Geometry check sheet. Reference: drawing and pictorial views, mm from the part's lowest x, y, z. A direction names the side the tool comes from. Round coordinates to 2 decimals unless told otherwise and drop trailing zeros. Write each loop counter-clockwise with the first axis right and the second up, starting at its lowest first coordinate (ties: lowest second). Pieces come first, ordered by that corner, then holes.
Item 1: Release check for a two-part mould opening along X. For the marked faces 1, 2 and 3 record: pulls with the +X half, pulls with the -X half, needs draft (parallel to the pull), parting line crosses it, or undercut.
Item 2: Section check D-D, the plane z = 16.75. Record the cut outline in (x, y).
Item 3: Section check A-A, the plane z = 9.75. State how many separate pieces and enclosed holes the cut face has, plus the area to 3 significant figures.
Item 4: Section check C-C, the plane x = 16. Record the cut outline in (y, z), plus the area to 3 significant figures.
Item 5: Depth check by flat-ended pin: pin 1 (1.5 mm diameter, centred on x = 11.5, y = 1, fed in from +Z); pin 2 (5.5 mm diameter, centred on x = 9.75, z = 9.75, fed in from -Y); pin 3 (4 mm diameter, centred on x = 2.75, z = 9.75, fed in from -Y). Enter the tip coordinate at first touch or a pass-through.
Item 6: Material ranges on line 1 along Z through (x, y) = (9.75, 4.2); line 2 along Z through (x, y) = (9.75, 3.85); line 3 along Y through (x, z) = (9.5, 12), recorded low to high.
Item 7: Set-up check for the marked faces 4 and 5: record each of +Z, -Z, +X, -X, +Y, -Y from which the full face is reachable in a straight line by a thin tool's end or side.
Item 8: Section check B-B, the plane x = 9. Record the cut outline in (y, z), plus the area to 3 significant figures.
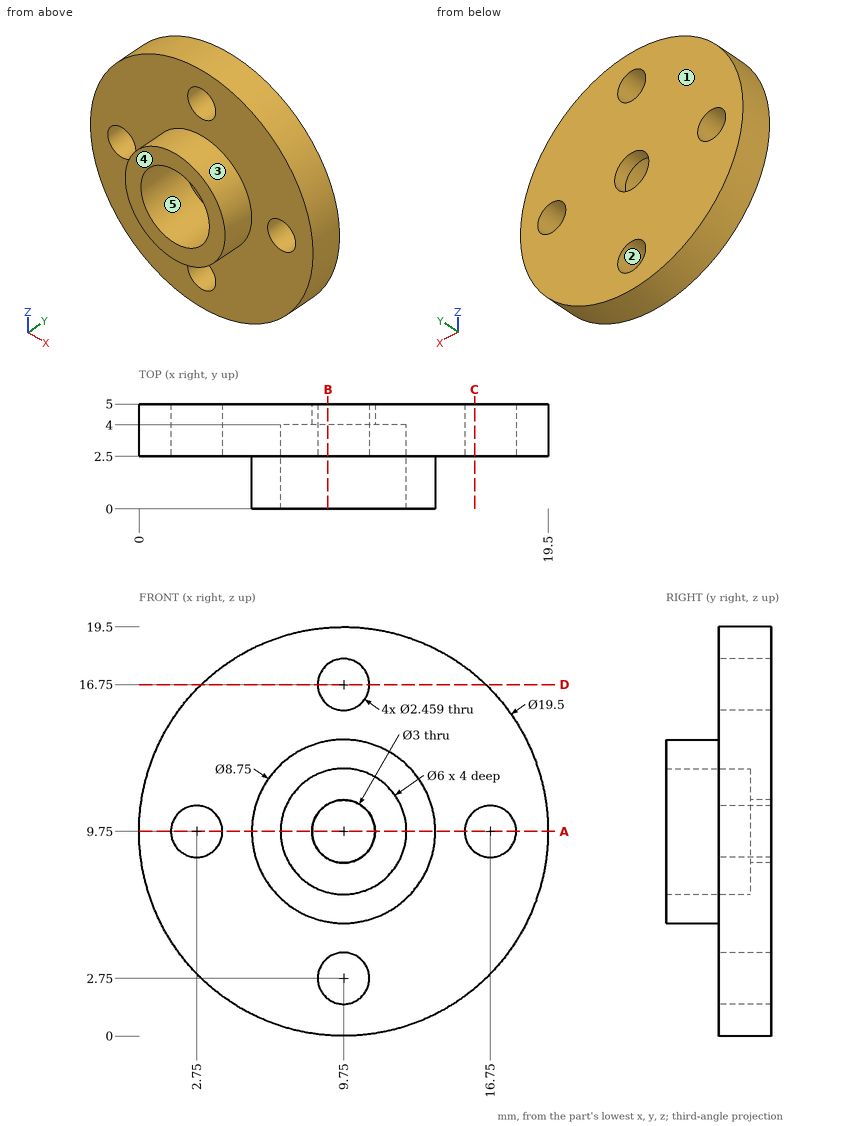
Values found:
1. face 1: needs draft
1. face 2: undercut
1. face 3: parting line crosses it
2. outline: (2.96, 2.5) - (8.52, 2.5) - (8.52, 5) - (2.96, 5) - close; (10.98, 2.5) - (16.54, 2.5) - (16.54, 5) - (10.98, 5) - close
3. separate pieces: 4
3. enclosed holes: 0
3. area: 31.3 mm2
4. outline: (2.5, 2.27) - (5, 2.27) - (5, 8.78) - (2.5, 8.78) - close; (2.5, 10.72) - (5, 10.72) - (5, 17.23) - (2.5, 17.23) - close
4. area: 32.5 mm2
5. pin 1: stops at z = 14.01
5. pin 2: stops at y = 4
5. pin 3: stops at y = 2.5
6. line 1: z = 0 to 1.52, 3.98 to 8.25, 11.25 to 15.52, 17.98 to 19.5
6. line 2: z = 0 to 1.52, 3.98 to 6.75, 12.75 to 15.52, 17.98 to 19.5
6. line 3: y = 4 to 5
7. face 4: +Z, -Z, +X, -X, -Y
7. face 5: -Y
8. outline: (0, 5.44) - (2.5, 5.44) - (2.5, 3.72) - (5, 3.72) - (5, 8.45) - (4, 8.45) - (4, 6.85) - (0, 6.85) - close; (0, 12.65) - (4, 12.65) - (4, 11.05) - (5, 11.05) - (5, 15.78) - (2.5, 15.78) - (2.5, 14.06) - (0, 14.06) - close; (2.5, 0.03) - (5, 0.03) - (5, 1.78) - (2.5, 1.78) - close; (2.5, 17.72) - (5, 17.72) - (5, 19.47) - (2.5, 19.47) - close
8. area: 34.6 mm2
